Build history of the part. All positions in model axes, mm. A direction names the side the tool comes from. Give positions to 0.01 mm unless a question says otherwise; leave off trailing zeros. Loops run counter-clockwise (first coordinate to the right, second up) from the corner with the lowest first, then second, coordinate; pieces in that order, holes last. Notation, with made-up numbers: M 13.25,-27.75 L 53.25,-27.75 A14 cw 53.25,-19.75 Z; hole C 53,-8 d9. An arc over 180 degrees is marked long. Answer in a Markdown table with one row per item. Add a question column.
```python
from build123d import *

# Parameters (mm, degrees)
SKETCH1_W           = 25
SKETCH1_H           = 25
BOSS_EXTRUDE1_DEPTH = 3
SKETCH2_W           = 20
SKETCH2_H           = 20
SKETCH2_R           = 5
CUT_EXTRUDE1_DEPTH  = 2
SKETCH3_R           = 1.25
CUT_EXTRUDE2_DEPTH  = 2


with BuildPart() as part:
    # Sketch1 → Boss-Extrude1 (new body)
    with BuildSketch(Plane(origin=(0, 0, 0), x_dir=(1, 0, 0), z_dir=(0, 1, 0))):
        Rectangle(SKETCH1_W, SKETCH1_H)
    extrude(amount=BOSS_EXTRUDE1_DEPTH)

    # Sketch2 → Cut-Extrude1 (cut)
    with BuildSketch(Plane.XZ):
        Rectangle(SKETCH2_W, SKETCH2_H)
        Circle(SKETCH2_R, mode=Mode.SUBTRACT)
    extrude(amount=-CUT_EXTRUDE1_DEPTH, mode=Mode.SUBTRACT)

    # Sketch3 → Cut-Extrude2 (cut)
    with BuildSketch(Plane.XZ):
        with Locations((-11, 11)):
            Circle(SKETCH3_R)
        with Locations((11, 11)):
            Circle(SKETCH3_R)
        with Locations((11, -11)):
            Circle(SKETCH3_R)
        with Locations((-11, -11)):
            Circle(SKETCH3_R)
    extrude(amount=-CUT_EXTRUDE2_DEPTH, mode=Mode.SUBTRACT)


solid = part.part
```
(1) Slice it at C-C, the plane x = 3. Give the cut face in (y, z).
(2) Pull direction X, two halves, no side cores. Call faces 3 (the flat face through (12.5, 1, 0)), 4 (the flat face through (0, 1, 12.5)), 5 (the flat face through (-11, 2, 11)), 6 (the flat face through (-12.5, 1, 0)): +X half, -X half, draft (parallel to the pull), parting line (faces both ways), or undercut.
(3) Slice it at D-D, the plane x = 5.5. Give the cut face in (y, z), then the cut area to 3 significant figures.
(4) Wall check: line 1 (Z direction, x = -11, y = 1.5); line 2 (X direction, y = 0.6, z = 8.75); line 3 (X direction, y = 0.4, z = 3). Give the ranges that are in metal, low to high.
(5) Slice it at A-A, the plane y = 0.9. Give the cut face in (x, z).
(6) Pin check, flat tips, straight feed: pin 1 (5 mm diameter, centred on x = -8, z = -2.5, fed in from -Y); pin 2 (2 mm diameter, centred on x = -11, z = 11, fed in from -Y). Stop position of each tip, or through.
(7) Slice it at B-B, the plane z = -11. Give the cut face in (x, y), then the cut area to 3 significant figures.
(8) Tool access for faces 1 (the cylindrical face through (-11.921, 0.986, 11.845)), 2 (the flat face through (-0.1, 0, -10.2)): list every direction of +Z, -Z, +X, -X, +Y, -Y with a clear straight run to the whole face (end or side of a thin tool).
Solution:
| question | item | result |
|---|---|---|
| 1 | outline | M 0,-12.5 L 3,-12.5 L 3,12.5 L 0,12.5 L 0,10 L 2,10 L 2,4 L 0,4 L 0,-4 L 2,-4 L 2,-10 L 0,-10 Z |
| 2 | face 3 | +X half |
| 2 | face 4 | draft |
| 2 | face 5 | undercut |
| 2 | face 6 | -X half |
| 3 | outline | M 0,-12.5 L 3,-12.5 L 3,12.5 L 0,12.5 L 0,10 L 2,10 L 2,-10 L 0,-10 Z |
| 3 | area | 35.0 mm^2 |
| 4 | line 1 | -12.5 to -12.25, -9.75 to 9.75, 12.25 to 12.5 |
| 4 | line 2 | -12.5 to -10, 10 to 12.5 |
| 4 | line 3 | -12.5 to -10, -4 to 4, 10 to 12.5 |
| 5 | outline | M -12.5,-12.5 L 12.5,-12.5 L 12.5,12.5 L -12.5,12.5 Z; C 0,0 d10; hole C -11,-11 d2.5; hole C -11,11 d2.5; hole M -10,-10 L 10,-10 L 10,10 L -10,10 Z; hole C 11,-11 d2.5; hole C 11,11 d2.5 |
| 6 | pin 1 | y = 0 |
| 6 | pin 2 | y = 2 |
| 7 | outline | M -12.5,0 L -12.25,0 L -12.25,2 L -9.75,2 L -9.75,0 L 9.75,0 L 9.75,2 L 12.25,2 L 12.25,0 L 12.5,0 L 12.5,3 L -12.5,3 Z |
| 7 | area | 65.0 mm^2 |
| 8 | face 1 | -Y |
| 8 | face 2 | +Z, -Z, +X, -X, -Y |
